The model under review builds one solid part; all positions refer to its coordinate system, in mm. Round coordinates to 2 decimals unless told otherwise and drop trailing zeros. Loops run counter-clockwise (first coordinate to the right, second up) from the corner with the lowest first, then second, coordinate; pieces in that order, holes last. Notation, with made-up numbers: M -18.75,37.25 L 39.25,37.25 A28 cw 39.25,65.25 Z; hole C 12.25,86 d7. An arc over 180 degrees is marked long. Return JSON: item names as keys, results as strings. Group by question number.
Q1. Clearance check with flat-ended pins moving along their axes: pin 1 Ø3 at (x, z) = (-2.5, 224.5) entering from +Y; pin 2 Ø1.1 at (x, z) = (0, 200.17) entering from -Y. State where each tip first meets the part, or that it passes through.
Q2. Consider section A-A (z = 217). State the section outline as (x, y) points (3 decimals), and give its area (3 significant figures).
Q3. To check wall thickness, follow line 1 along Z through (x, y) = (0, -1.05); line 2 along Z through (x, y) = (-0.25, 1.5); line 3 along X through (y, z) = (0.25, 263). State the ranges of each line that lie inside material, in increasing order.
from build123d import *

# Parameters (mm, degrees)
SKETCH3_R               = 3.175
BOSS_EXTRUDE1_DEPTH     = 304.8
CHAMFER1_SIZE           = 0.635
CUT_EXTRUDE1_START      = -106.219625
SKETCH4_R               = 3.175
CUT_EXTRUDE1_DEPTH      = 504.380375
SKETCH5_R               = 0.5953125
CUT_EXTRUDE2_DEPTH      = 4.175
CUT_EXTRUDE2_DEPTH_BACK = 4.175


with BuildPart() as part:
    # Sketch3 → Boss-Extrude1 (new body, symmetric)
    with BuildSketch(Plane.XY):
        Circle(SKETCH3_R)
    extrude(amount=BOSS_EXTRUDE1_DEPTH, both=True)

    # Chamfer1
    chamfer1_edges = [part.edges().sort_by_distance(p)[0] for p in [
        (-3.175, 0, -304.8),
        (-3.175, 0, 304.8),
    ]]
    chamfer(chamfer1_edges, length=CHAMFER1_SIZE)

    # Sketch4 → Cut-Extrude1 (cut, through all)
    with BuildSketch(Plane.XY.offset(304.8).offset(CUT_EXTRUDE1_START)):
        Circle(SKETCH4_R)
    extrude(amount=-CUT_EXTRUDE1_DEPTH, mode=Mode.SUBTRACT)

    # Sketch5 → Cut-Extrude2 (cut, two sides)
    with BuildSketch(Plane(origin=(0, 0, 0), x_dir=(1, 0, 0), z_dir=(0, 1, 0))) as cut_extrude2_sk:
        with Locations((0, -200.167875)):
            Circle(SKETCH5_R)
        with Locations((0, -303.2125)):
            Circle(SKETCH5_R)
    extrude(amount=CUT_EXTRUDE2_DEPTH, mode=Mode.SUBTRACT)
    extrude(cut_extrude2_sk.sketch, amount=-CUT_EXTRUDE2_DEPTH_BACK, mode=Mode.SUBTRACT)


solid = part.part
Values:
{
 "1": {"pin 1": "stops at y = 3.01", "pin 2": "passes through"},
 "2": {"outline": "C 0,0 d6.35", "area": "31.7 mm2"},
 "3": {"line 1": "z = 198.58 to 199.57, 200.76 to 302.62, 303.81 to 304.8", "line 2": "z = 198.58 to 199.63, 200.71 to 302.67, 303.75 to 304.8", "line 3": "x = -3.17 to 3.17"}
}
